from build123d import *

# Parameters (mm, degrees)
F1_R = 2.1902863251
F4_R = 2.8180913068


with BuildPart() as f2:
    # F2: sweep along a path in F0
    with BuildLine(Plane.XZ) as f2_path:
        CenterArc((0, 0), 19.2595042625, 0, 360)
    # F1 (on Right) → F2 (sweep)
    with BuildSketch(Plane.YZ):
        with Locations((0, 19.164359197)):
            Circle(F1_R)
    sweep(path=f2_path.line)

    # F5: sweep along a path in F3
    with BuildLine(Plane.XZ) as f5_path:
        Line((-8.6774716492, 27.7112331241), (-17.3549432985, 42.7410549019))
        Line((-17.3549432985, 42.7410549019), (-8.6774716492, 57.7708766796))
        Line((-8.6774716492, 57.7708766796), (8.6774716492, 57.7708766796))
        Line((8.6774716492, 57.7708766796), (17.3549432985, 42.7410549019))
        Line((17.3549432985, 42.7410549019), (8.6774716492, 27.7112331241))
        Line((8.6774716492, 27.7112331241), (-8.6774716492, 27.7112331241))
    # F4 (on Right) → F5 (sweep)
    with BuildSketch(Plane.YZ):
        with Locations((0, 61.8414543569)):
            Circle(F4_R)
    sweep(path=f5_path.line, transition=Transition.RIGHT)


solid = f2.part
Read the model definition and answer for the solid it produces. Units are mm, in the model's axes. Round coordinates to 2 decimals unless told otherwise and drop trailing zeros. Write each loop counter-clockwise with the first axis right and the second up, starting at its lowest first coordinate (ties: lowest second). Pieces come first, ordered by that corner, then holes.
Q1. Find section B-B on x = 17.5. State how many separate pieces and enclosed holes the cut face has, and give its area (3 significant figures).
Values:
separate pieces: 3
enclosed holes: 0
area: 187 mm2
Q2. Flat-ended cylindrical pins translate along their axes: P1, Ø3, axis at x = -16, y = -2, coming from the +Z side; P2, Ø3, axis at y = 0, z = 24.5, coming from the +X side; P3, Ø1.5, axis at y = -2, z = 42, coming from the -X side; P4, Ø6, axis at x = -7, z = 21.5, coming from the -Y side. Find the tip coordinate at first contact, or state that the pin passes through.
Values:
P1: stops at z = 60.53
P2: stops at x = 15.64
P3: stops at x = -24.71
P4: stops at y = -2.82
Q3. Straight lines are drawn through the part: line 1 (Z direction, x = -5.5, y = 2); line 2 (Z direction, x = 13, y = 0.1); line 3 (Z direction, x = -18, y = 0.8). For each, find the intervals that lie inside material, in ascending order.
Values:
line 1: z = -19.29 to -17.42, 17.42 to 19.29, 21.66 to 25.63, 59.86 to 63.83
line 2: z = -16.94 to -10.92, 10.92 to 16.94, 21.42 to 32.69, 52.79 to 64.06
line 3: z = -11.21 to 11.21, 30.31 to 41.12, 44.36 to 55.17
Q4. Find section A-A on y = -0.95. Determine the outline of the cut face in (x, z), and give its area (3 significant figures).
Values:
outline: (-25.12, 42.74) - (-12.56, 20.99) - (-2.52, 20.99) arc R21.14 ccw (long way) to (2.52, 20.99) - (12.56, 20.99) - (25.12, 42.74) - (12.56, 64.49) - (-12.56, 64.49) - close; hole (-18.99, 42.74) - (-9.5, 26.29) - (9.5, 26.29) - (18.99, 42.74) - (9.5, 59.19) - (-9.5, 59.19) - close; hole circle Ø34.38 at (0, 0)
area: 1,180 mm2
